Geometry check sheet. Reference: the model listing, model coordinates, mm. A direction names the side the tool comes from. Give positions to 0.01 mm unless a question says otherwise; leave off trailing zeros. Loops run counter-clockwise (first coordinate to the right, second up) from the corner with the lowest first, then second, coordinate; pieces in that order, holes last. Notation, with made-up numbers: (31.5, 30) -> (53.5, 30) arc R3 cw to (53.5, 34) -> close; hole circle Ø3 at (30, -19.75). An arc over 180 degrees is marked (long way). One line per item, written item: value. Start each with the question number.
(1) Scan lines: line 1 along Y through (x, z) = (57.8, -56); line 2 along Y through (x, z) = (-3, -21.5); line 3 along X through (y, z) = (11.5, -50.5). Record each from-to range of solid material in increasing order. Write a range as from..to.
(2) Gauge pin test, flat ends, axial feed: pin 1 Ø2.5 at (x, y) = (-57.8, 12.05) entering from +Z; pin 2 Ø3 at (x, y) = (-6.5, -12) entering from -Z; pin 3 Ø12 at (x, y) = (-12.5, 1) entering from -Z. Record the tip position at first contact, or that the pin passes through.
(3) Sectioned sample at C-C, the plane x = -38. Record the cut outline in (y, z).
(4) Draft check along Y on faces 4 (the face through (-60.981, 15.162, -65.91)), 5 (the face through (0, -13, -128.5)), 6 (the face through (-62.25, 0, -64)). Enter one of: pulls with the +Y half, pulls with the -Y half, needs draft (parallel to the pull), parting line crosses it, or undercut.
(5) Sectioned sample at A-A, the plane y = -1.5. Record the cut outline in (x, z).
(6) Tool access check on faces 1 (the face through (-40, -14.05, -64)), 2 (the face through (-59, -13, -1.5)), 3 (the face through (59, 13, -128.5)). Record the directions out of +Z, -Z, +X, -X, +Y, -Y that give a thin tool (end or side, any length) a straight path to the whole face; none if there is none.
(7) Sectioned sample at B-B, the plane x = -1. Record the cut outline in (y, z).
(8) Sectioned sample at D-D, the plane z = -35. State how many separate pieces and enclosed holes the cut face has, then the cut area to 3 significant figures.
Autodesk Inventor part; units mm, degrees
ref_plane "YZ Plane" through (0, 0, 0) normal (1, 0, 0) x (0, 1, 0)
ref_plane "XZ Plane" through (0, 0, 0) normal (0, 1, 0) x (-1, 0, 0)
ref_plane "XY Plane" through (0, 0, 0) normal (0, 0, 1) x (1, 0, 0)
sketch "Sketch1" plane through (0, 0, 0) normal (0, 0, 1) x (1, 0, 0)
  line L0 (-62.25, 16.5) -> (62.25, 16.5)
  line L1 (62.25, 16.5) -> (62.25, -16.5)
  line L2 (62.25, -16.5) -> (-62.25, -16.5)
  line L3 (-62.25, -16.5) -> (-62.25, 16.5)
  line L4 (-60.25, 14.5) -> (60.25, 14.5)
  line L5 (60.25, 14.5) -> (60.25, -14.5)
  line L6 (60.25, -14.5) -> (-60.25, -14.5)
  line L7 (-60.25, -14.5) -> (-60.25, 14.5)
  point P0 (0, 0)
  dimension "d0" = 124.5
  dimension "d1" = 62.25
  dimension "d2" = 120.5
  dimension "d3" = 60.25
  dimension "d4" = 33
  dimension "d5" = 29
  dimension "d6" = 16.5
  dimension "d7" = 14.5
extrude "Extrusion1" add sketch "Sketch1" against normal blind 130
sketch "Sketch2" plane through (0, 0, 0) normal (0, 0, 1) x (1, 0, 0)
  line L0 (60.25, -14.5) -> (-60.25, -14.5)
  line L1 (-15.935, -14.5) -> (15.935, -14.5)
  line L2 (15.935, -14.5) -> (15.935, -10.95)
  line L3 (15.935, -10.95) -> (-15.935, -10.95)
  line L4 (-15.935, -10.95) -> (-15.935, -14.5)
  point P0 (0, 0)
  dimension "d10" = 31.87
  dimension "d11" = 15.935
  dimension "d12" = 3.55
extrude "Extrusion2" add sketch "Sketch2" against normal blind 130
chamfer "Chamfer1" distance 3.55 angle 45 2 edges at (15.935, -14.5, -65) (-15.935, -14.5, -65)
sketch "Sketch3" plane through (0, 0, 0) normal (0, 0, 1) x (1, 0, 0)
  line L0 (-19.485, -14.5) -> (-60.25, -14.5)
  line L1 (-45.4675, -14.5) -> (-34.2675, -14.5)
  line L2 (-34.2675, -14.5) -> (-34.2675, -14.05)
  line L3 (-34.2675, -14.05) -> (-45.4675, -14.05)
  line L4 (-45.4675, -14.05) -> (-45.4675, -14.5)
  line L5 (-60.25, 14.5) -> (-60.25, -14.5)
  point P0 (0, 0)
  point P1 (-60.25, -14.5)
  dimension "d18" = 40.765
  dimension "d19" = 11.2
  dimension "d20" = 0.45
  dimension "d21" = 14.7825
  dimension "d22" = 14.7825
extrude "Extrusion3" add sketch "Sketch3" against normal blind 130
chamfer "Chamfer2" distance 0.45 angle 45 2 edges at (-45.4675, -14.5, -65) (-34.2675, -14.5, -65)
sketch "Sketch4" plane through (0, 0, 0) normal (0, 0, 1) x (1, 0, 0)
  line L0 (60.25, -14.5) -> (19.485, -14.5)
  line L1 (34.2675, -14.5) -> (45.4675, -14.5)
  line L2 (45.4675, -14.5) -> (45.4675, -14.05)
  line L3 (45.4675, -14.05) -> (34.2675, -14.05)
  line L4 (34.2675, -14.05) -> (34.2675, -14.5)
  point P0 (0, 0)
  dimension "d28" = 11.2
  dimension "d29" = 0.45
  dimension "d30" = 14.7825
extrude "Extrusion4" add sketch "Sketch4" against normal blind 130
chamfer "Chamfer3" distance 0.45 angle 45 2 edges at (34.2675, -14.5, -65) (45.4675, -14.5, -65)
sketch "Sketch5" plane through (0, 0, 0) normal (0, 0, 1) x (1, 0, 0)
  circle A0 centre (-57.8, 12.05) radius 2
  circle A1 centre (57.8, 12.05) radius 2
  line L0 (62.25, -16.5) -> (62.25, 16.5)
  line L1 (62.25, 16.5) -> (-62.25, 16.5)
  line L2 (-62.25, 16.5) -> (-62.25, -16.5)
  line L3 (-60.25, 14.5) -> (-60.25, -14.5)
  line L4 (-57.8, 10.05) -> (-60.25, 10.05)
  line L5 (-60.25, 10.05) -> (-60.25, 14.5)
  line L6 (-60.25, 14.5) -> (-57.8, 14.5)
  line L7 (-57.8, 14.5) -> (-57.8, 10.05)
  line L8 (-57.8, 14.5) -> (-57.2, 14.5)
  line L9 (-57.2, 14.5) -> (-57.2, 13.9579)
  line L10 (-57.2, 13.9579) -> (-57.8, 13.9579)
  line L11 (-57.8, 13.9579) -> (-57.8, 14.5)
  line L12 (60.25, 14.5) -> (-60.25, 14.5)
  line L13 (60.25, 14.5) -> (57.8, 14.5)
  line L14 (57.8, 14.5) -> (57.8, 10.05)
  line L15 (57.8, 10.05) -> (60.25, 10.05)
  line L16 (60.25, 10.05) -> (60.25, 14.5)
  line L17 (57.8, 14.5) -> (57.2, 14.5)
  line L18 (57.2, 14.5) -> (57.2, 13.9579)
  line L19 (57.2, 13.9579) -> (57.8, 13.9579)
  line L20 (57.8, 13.9579) -> (57.8, 14.5)
  circle A2 centre (-57.8, -12.05) radius 2
  circle A3 centre (57.8, -12.05) radius 2
  line L21 (-62.25, -16.5) -> (62.25, -16.5)
  line L22 (-57.8, -10.05) -> (-60.25, -10.05)
  line L23 (-60.25, -10.05) -> (-60.25, -14.5)
  line L24 (-60.25, -14.5) -> (-57.8, -14.5)
  line L25 (-57.8, -14.5) -> (-57.8, -10.05)
  line L26 (60.25, 14.5) -> (60.25, -14.5)
  line L27 (57.8, -10.05) -> (60.25, -10.05)
  line L28 (60.25, -10.05) -> (60.25, -14.5)
  line L29 (60.25, -14.5) -> (57.8, -14.5)
  line L30 (57.8, -14.5) -> (57.8, -10.05)
  line L31 (57.2, -13.9579) -> (57.8, -13.9579)
  line L32 (57.8, -13.9579) -> (57.8, -14.5)
  line L33 (57.8, -14.5) -> (57.2, -14.5)
  line L34 (57.2, -14.5) -> (57.2, -13.9579)
  line L35 (-57.8, -14.5) -> (-57.0401, -14.5)
  line L36 (-57.0401, -14.5) -> (-57.0401, -13.9)
  line L37 (-57.0401, -13.9) -> (-57.8, -13.9)
  line L38 (-57.8, -13.9) -> (-57.8, -14.5)
  point P0 (0, 0)
  point P1 (-55.8, 12.05)
  point P2 (55.8, 12.05)
  dimension "d36" = 115.6
  dimension "d37" = 4.45
  dimension "d38" = 4.45
  dimension "d39" = 4.45
  dimension "d40" = 4.45
  dimension "d41" = 111.6
  dimension "d42" = 4
  dimension "d43" = 4
  dimension "d44" = 0.6
  dimension "d45" = 4.45
  dimension "d46" = 4.45
  dimension "d47" = 0.6
  dimension "d48" = 4
  dimension "d49" = 4.45
  dimension "d50" = 4.45
  dimension "d51" = 4.45
  dimension "d52" = 4.45
  dimension "d53" = 0.6
  dimension "d54" = 4.45
  dimension "d55" = 4
  dimension "d56" = 0.6
extrude "Extrusion5" add sketch "Sketch5" against normal blind 130 contours A0 L7 L10 | L22 A2 L25 L24 L3 | L26 L29 L30 A3 L27 | L12 L14 A1 L18 | L10 L7 A0 | A0 L7 L8 L9 | L4 L3 L6 L7 A0 | A0 L7 | L12 L16 L15 A1 L14 | L19 L14 A1 | A1 L14 L19 | L25 A2 | A2 L37 L25 | A1 L14 | L25 A2 L36 L35 | L25 L37 A2 | L30 L31 A3 | A3 L30 | L33 L34 A3 L30 | L31 L30 A3
sketch "Sketch6" plane through (0, 0, 0) normal (0, 0, 1) x (1, 0, 0)
  arc A0 (-57.8, 10.05) -> (-57.2, 13.9579) centre (-57.8, 12.05) ccw
  arc A1 (-57.0401, -13.9) -> (-57.8, -10.05) centre (-57.8, -12.05) ccw
  arc A2 (57.8, -10.05) -> (57.2, -13.9579) centre (57.8, -12.05) ccw
  arc A3 (57.2, 13.9579) -> (57.8, 10.05) centre (57.8, 12.05) ccw
  circle A4 centre (-57.8, 12.05) radius 1
  circle A5 centre (-57.8, -12.05) radius 1
  circle A6 centre (57.8, -12.05) radius 1
  circle A7 centre (57.8, 12.05) radius 1
  point P0 (0, 0)
  dimension "d59" = 2
  dimension "d60" = 2
  dimension "d61" = 2
  dimension "d62" = 2
extrude "Extrusion6" cut sketch "Sketch6" against normal blind 130
fillet "Fillet1" radius 4.45 4 edges at (-62.25, 16.5, -65) (-62.25, -16.5, -65) (62.25, -16.5, -65) (62.25, 16.5, -65)
sketch "Sketch7" plane through (0, 0, 0) normal (0, 0, 1) x (1, 0, 0)
  line L0 (-60.25, 14.5) -> (60.25, 14.5)
  line L1 (60.25, 14.5) -> (60.25, -14.5)
  line L2 (60.25, -14.5) -> (-60.25, -14.5)
  line L3 (-60.25, -14.5) -> (-60.25, 14.5)
  line L4 (-57.2, 14.5) -> (57.2, 14.5)
  line L5 (60.25, 10.05) -> (60.25, -10.05)
  line L6 (33.8175, -14.5) -> (19.485, -14.5)
  line L7 (-60.25, -10.05) -> (-60.25, 10.05)
  arc A0 (-57.8, 10.05) -> (-57.2, 13.9579) centre (-57.8, 12.05) ccw
  circle A1 centre (-57.8, 12.05) radius 2.45
  arc A2 (-57.0401, -13.9) -> (-57.8, -10.05) centre (-57.8, -12.05) ccw
  circle A3 centre (-57.8, -12.05) radius 2.45
  circle A4 centre (57.8, -12.05) radius 1
  circle A5 centre (57.8, -12.05) radius 2.45
  circle A6 centre (57.8, 12.05) radius 1
  circle A7 centre (57.8, 12.05) radius 2.45
  point P0 (0, 0)
  point P1 (57.8, 14.5)
  point P2 (-57.8, 14.5)
  point P3 (-60.25, 12.05)
  point P4 (-60.25, -12.05)
  point P5 (-57.8, -14.5)
  point P6 (57.8, -14.5)
  point P7 (60.25, -12.05)
  point P8 (60.25, 12.05)
extrude "Extrusion7" cut sketch "Sketch7" against normal blind 1.5 contours L0 A7 L1 A5 L2 A3 L3 A1 | A1 | A7 | A3 | A5 | A4 | A6
sketch "Sketch8" plane through (0, 0, -130) normal (0, 0, -1) x (-1, 0, 0)
  line L0 (-60.25, 14.5) -> (60.25, 14.5)
  line L1 (60.25, 14.5) -> (60.25, -14.5)
  line L2 (60.25, -14.5) -> (-60.25, -14.5)
  line L3 (-60.25, -14.5) -> (-60.25, 14.5)
  line L4 (-57.2, 14.5) -> (57.2, 14.5)
  line L5 (60.25, 10.05) -> (60.25, -10.05)
  line L6 (33.8175, -14.5) -> (19.485, -14.5)
  line L7 (-60.25, -10.05) -> (-60.25, 10.05)
  circle A0 centre (-57.8, 12.05) radius 1
  circle A1 centre (-57.8, 12.05) radius 2.45
  line L8 (57.8, 14.5) -> (-57.8, 14.5)
  circle A2 centre (-57.8, -12.05) radius 1
  circle A3 centre (-57.8, -12.05) radius 2.45
  circle A4 centre (57.8, -12.05) radius 1
  line L9 (-57.8, -14.5) -> (57.8, -14.5)
  circle A5 centre (57.8, -12.05) radius 2.45
  circle A6 centre (57.8, 12.05) radius 1
  circle A7 centre (57.8, 12.05) radius 2.45
  point P0 (0, 0)
  point P1 (-60.25, 12.05)
  point P2 (-60.25, -12.05)
  point P3 (-57.8, -14.5)
  point P4 (60.25, -12.05)
  point P5 (60.25, 12.05)
extrude "Extrusion8" cut sketch "Sketch8" against normal blind 1.5 contours L0 A7 L1 A5 L2 A3 L3 A1 | A1 | A7 | A3 | A5 | A0 | A2 | A4 | A6
properties part number "case_dummy"
Calculated:
1. line 1: y = -16.5..-13.05, -11.05..-10.05, 10.05..11.05, 13.05..16.5
1. line 2: y = -16.5..-10.95, 14.5..16.5
1. line 3: x = -62.25..-58.64, -56.96..-55.88, 55.88..56.96, 58.64..62.25
2. pin 1: stops at z = -1.5
2. pin 2: stops at z = -128.5
2. pin 3: passes through
3. outline: (-16.5, -130) -> (-14.5, -130) -> (-14.5, -128.5) -> (-14.05, -128.5) -> (-14.05, -1.5) -> (-14.5, -1.5) -> (-14.5, 0) -> (-16.5, 0) -> close; (14.5, -130) -> (16.5, -130) -> (16.5, 0) -> (14.5, 0) -> close
4. face 4: pulls with the +Y half
4. face 5: undercut
4. face 6: needs draft
5. outline: (-62.25, -130) -> (-60.25, -130) -> (-60.25, 0) -> (-62.25, 0) -> close; (60.25, -130) -> (62.25, -130) -> (62.25, 0) -> (60.25, 0) -> close
6. face 1: +Z, -Z
6. face 2: +Z
6. face 3: -Z
7. outline: (-16.5, -130) -> (-14.5, -130) -> (-14.5, -128.5) -> (-10.95, -128.5) -> (-10.95, -1.5) -> (-14.5, -1.5) -> (-14.5, 0) -> (-16.5, 0) -> close; (14.5, -130) -> (16.5, -130) -> (16.5, 0) -> (14.5, 0) -> close
8. separate pieces: 1
8. enclosed holes: 5
8. area: 791 mm2
